Geometry check sheet. Reference: drawing and pictorial views, mm from the part's lowest x, y, z. A direction names the side the tool comes from. Coordinates: 2 decimals unless noted, no trailing zeros. Order: outer loops, then holes, each group sorted by start corner. A loop starts at its lowest first (then second) coordinate and runs counter-clockwise, first axis right, second up. Notation, with made-up numbers: (60.25, -0.5) -> (64.25, -0.5) arc R23 cw to (64.25, 31.5) -> close; hole circle Ø1 at (-1, 67). An arc over 180 degrees is marked (long way). Use CSV: the item, a comma, the result in double quotes. Start each with the question number.
1) Go/stop test with flat-tipped pins: pin 1 (3 mm diameter, centred on x = 7.5, z = 9, fed in from -Y); pin 2 (4 mm diameter, centred on y = 17, z = 7, fed in from +X). Record where each tip stops, or that it passes through.
2) Sectioned sample at D-D on z = 9.75. Give the number of separate pieces and of enclosed holes in the cut face, then the cut area to 3 significant figures.
3) Release check for a two-part mould opening along Y. For the marked faces 4, 5 and 6 record: released by +Y, released by -Y, zero draft, split by the parting line, or undercut.
4) Tool access check on the marked faces 1, 2 and 3. Record the directions out of +Z, -Z, +X, -X, +Y, -Y that give a thin tool (end or side, any length) a straight path to the whole face; none if there is none.
5) Scan lines: line 1 along Z through (x, y) = (7, 3); line 2 along Y through (x, z) = (5, 7); line 3 along Z through (x, y) = (8.5, 13). Record each from-to range of solid material in increasing order.
6) Sectioned sample at B-B on x = 7.5. Record the boundary of the cut face in (y, z), then the cut area to 3 significant figures.
7) Sectioned sample at C-C on y = 3. Record the boundary of the cut face in (x, z).
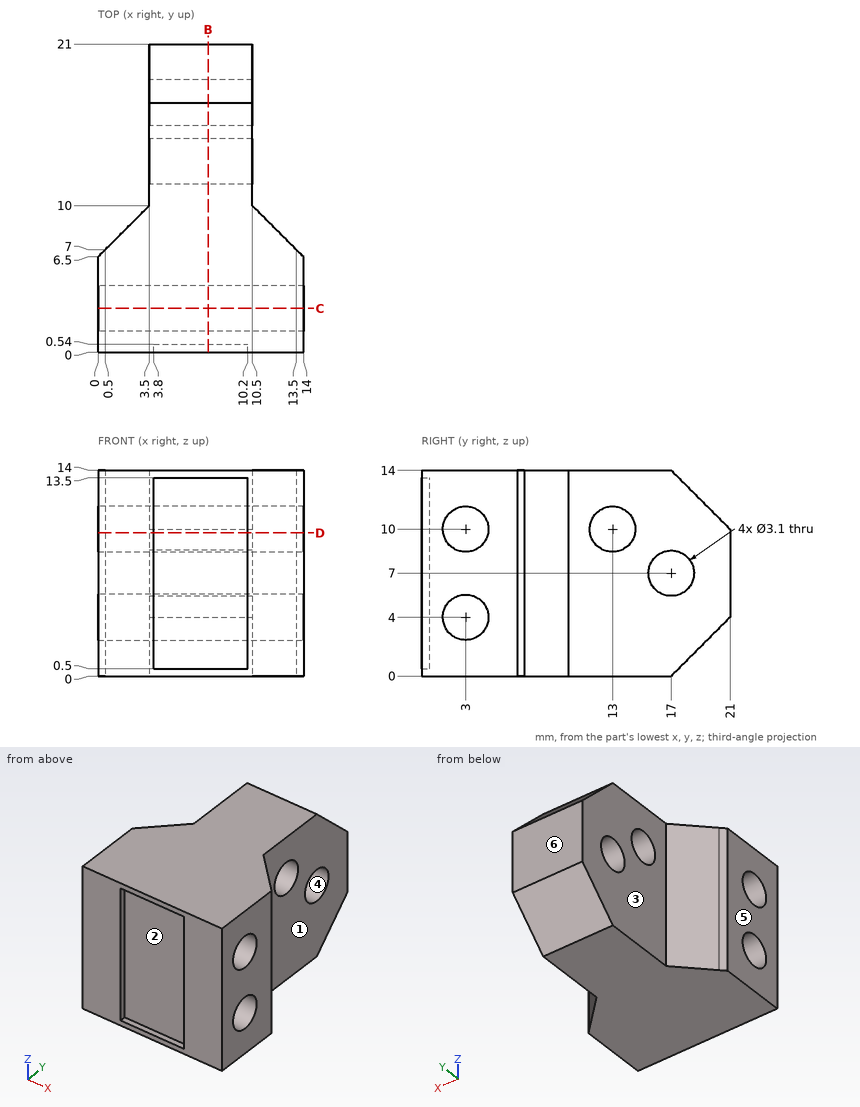
Answers follow:
1,pin 1,"stops at y = 0.54"
1,pin 2,"stops at x = 10.5"
2,separate pieces,"3"
2,enclosed holes,"0"
2,area,"137 mm²"
3,face 4,"undercut"
3,face 5,"zero draft"
3,face 6,"released by +Y"
4,face 1,"+Z, -Z, +X, +Y"
4,face 2,"-Y"
4,face 3,"+Z, -Z, -X, +Y"
5,line 1,"z = 0 to 2.45, 5.55 to 8.45, 11.55 to 14"
5,line 2,"y = 0.54 to 15.45, 18.55 to 21"
5,line 3,"z = 0 to 8.45, 11.55 to 14"
6,outline,"(0, 0) -> (17, 0) -> (21, 4) -> (21, 10) -> (17, 14) -> (0, 14) -> (0, 13.5) -> (0.54, 13.5) -> (0.54, 0.5) -> (0, 0.5) -> close; hole circle Ø3.1 at (3, 4); hole circle Ø3.1 at (3, 10); hole circle Ø3.1 at (13, 10); hole circle Ø3.1 at (17, 7)"
6,area,"241 mm²"
7,outline,"(0, 0) -> (14, 0) -> (14, 2.45) -> (0, 2.45) -> close; (0, 5.55) -> (14, 5.55) -> (14, 8.45) -> (0, 8.45) -> close; (0, 11.55) -> (14, 11.55) -> (14, 14) -> (0, 14) -> close"
